```python
from build123d import *

# Parameters (mm, degrees)
F0_W     = 88
F0_H     = 88
F1_DEPTH = 1700
F3_DEPTH = 31
F5_DEPTH = 31
F7_DEPTH = 88.001
F9_DEPTH = 88.001
F10_R    = 5


with BuildPart() as f1:
    # F0 (on Top) → F1 (new body)
    with BuildSketch(Plane.XY):
        with Locations((44, 44)):
            Rectangle(F0_W, F0_H)
    extrude(amount=F1_DEPTH)

    # F2 (on face) → F3 (cut)
    with BuildSketch(Plane.YZ.offset(88)):
        Polygon((29, 282), (44, 282), (59, 282), (59, 370), (29, 370), align=None)
    extrude(amount=-F3_DEPTH, mode=Mode.SUBTRACT)

    # F4 (on face) → F5 (cut)
    with BuildSketch(Plane.YZ.offset(88)):
        Polygon((29, 1460), (44, 1460), (59, 1460), (59, 1548), (29, 1548), align=None)
    extrude(amount=-F5_DEPTH, mode=Mode.SUBTRACT)

    # F6 (on face) → F7 (cut, through all)
    with BuildSketch(Plane.YZ.offset(88)):
        Polygon((0, 1663.5492065112), (88, 1700), (0, 1700), align=None)
    extrude(amount=-F7_DEPTH, mode=Mode.SUBTRACT)

    # F8 (on face) → F9 (cut, through all)
    with BuildSketch(Plane.YZ.offset(88)):
        Polygon((23, 1594.0761184457), (23, 1673.0761184457), (0, 1663.5492065112), (0, 1584.5492065112), align=None)
    extrude(amount=-F9_DEPTH, mode=Mode.SUBTRACT)

    # F10
    f10_edges = [f1.edges().sort_by_distance(p)[0] for p in [
        (0, 0, 792.274603),
        (88, 0, 792.274603),
        (88, 88, 850),
        (0, 88, 850),
    ]]
    fillet(f10_edges, radius=F10_R)


solid = f1.part
```
For this review, take the finished solid that the model builds, in its own axes (mm). A direction names the side the tool comes from. Coordinates: 2 decimals unless noted, no trailing zeros. Write each loop counter-clockwise with the first axis right and the second up, starting at its lowest first coordinate (ties: lowest second). Pieces come first, ordered by that corner, then holes. Notation, with made-up numbers: (-37.75, 31) - (-4.75, 31) arc R8 ccw to (-4.75, 44) - close; hole circle Ø7 at (70, -30). An arc over 180 degrees is marked (long way). Answer in a Markdown table with one row per item. Add a question column.
Q1. For P1, Ø15, axis at x = 77.5, y = 43, coming from the +Z side; P2, Ø9, axis at x = 69.5, y = 51, coming from the +Z side; P3, Ø10, axis at x = 77.5, y = 34.5, coming from the +Z side, all flat-tipped, find the tip position at first contact; note any pin that passes through.
Q2. For probe 1 along Y at (x, z) = (63, 1502.5); probe 2 along X at (y, z) = (33, 298.5); probe 3 along Y at (x, z) = (4.5, 161), list the stretches that pass through material, from the lowest coordinate up.
Q3. We need section A-A, the plane z = 1514.5. State the section outline as (x, y) points, and give its area (3 significant figures).
Q4. We need section B-B, the plane x = 23.5. State the section outline as (y, z) points, and give its area (3 significant figures).
Q5. Tool access review of faces 4 (the flat face through (0, 43, 837)), 5 (the flat face through (45, 23, 1633)), 6 (the flat face through (57, 44, 1505)): name each direction out of +Z, -Z, +X, -X, +Y, -Y from which nothing blocks a thin tool from reaching the whole face with its end or side.
Q6. Draft analysis for pull direction Z (two halves, no side actions). For faces 1 (the flat face through (73, 29, 327)), 2 (the flat face through (43, 45, 0)), 3 (the flat face through (88, 43, 837)), state which applies: +Z half, -Z half, draft (parallel to the pull), parting line (faces both ways), or undercut.
Answer list:
| question | item | result |
|---|---|---|
| 1 | P1 | stops at z = 1684.47 |
| 1 | P2 | stops at z = 1686.54 |
| 1 | P3 | stops at z = 1679.91 |
| 2 | probe 1 | y = 0 to 29, 59 to 88 |
| 2 | probe 2 | x = 0 to 57 |
| 2 | probe 3 | y = 0.03 to 87.97 |
| 3 | outline | (0, 5) arc R5 ccw to (5, 0) - (83, 0) arc R5 ccw to (88, 5) - (88, 29) - (57, 29) - (57, 59) - (88, 59) - (88, 83) arc R5 ccw to (83, 88) - (5, 88) arc R5 ccw to (0, 83) - close |
| 3 | area | 6,790 mm2 |
| 4 | outline | (0, 0) - (88, 0) - (88, 1700) - (23, 1673.08) - (23, 1594.08) - (0, 1584.55) - close |
| 4 | area | 146,000 mm2 |
| 5 | face 4 | +Z, -Z, -X, +Y, -Y |
| 5 | face 5 | +Z, +X, -X, -Y |
| 5 | face 6 | +X |
| 6 | face 1 | undercut |
| 6 | face 2 | -Z half |
| 6 | face 3 | draft |
